Source: CAD feature listing. Evaluate the final solid. Frame: model axes, mm. Face numbers are marked on the shaded views. A direction names the side the tool comes from. Round coordinates to 2 decimals unless told otherwise and drop trailing zeros. Order: outer loops, then holes, each group sorted by start corner. A loop starts at its lowest first (then second) coordinate and runs counter-clockwise, first axis right, second up. Notation, with made-up numbers: (86, 51) -> (98, 51) arc R16 cw to (98, 62) -> close; hole circle Ø2 at (46, 49). An arc over 180 degrees is marked (long way). Answer as CSV lines item,"result". Start each with the question number.
(1) Line query: line 1 along Z through (x, y) = (-8, 6); line 2 along X through (y, z) = (40.5, -2.75); line 3 along Z through (x, y) = (20.5, 46.5). Output: solid intervals per line, ascending. Write a range as from..to.
(2) Section query A-A (x = -17). Output: boundary loops of the cut face in (y, z).
(3) Pull-direction query (Z, two-part tool) for the marked faces 3, 4 and 5; classes: +Z half, -Z half, draft (parallel to the pull), parting line (faces both ways), or undercut.
(4) Section query B-B (z = 5.5). Output: boundary loops of the cut face in (x, y), plus the area to 3 significant figures.
(5) Section query C-C (y = 75.5). Output: boundary loops of the cut face in (x, z) (3 decimals).
(6) Set-up query: the marked faces 1 and 2. Return all of +Z, -Z, +X, -X, +Y, -Y with unobstructed straight access to the full face (end or side cutting, diameter ignored); none if empty.
(7) Contact query for a flat-ended pin moving along its axis: P1, Ø3, axis at y = 50, z = -9, coming from the +X side. Output: stop coordinate, or through.
Solid Edge part; units mm, degrees
sketch "Sketch1" plane through (0, 0, 0) normal (1, 0, 0) x (0, 1, 0)
  line L0 (0, 0) -> (127.0003, 0)
sketch "Sketch2" plane through (0, 0, 0) normal (0, -1, 0) x (1, 0, 0)
  line L0 (25.4001, -6.985) -> (25.4001, 6.985)
  arc A0 (19.6851, 12.7) -> (25.4001, 6.985) centre (19.6851, 6.985) cw
  line L1 (19.6851, 12.7) -> (-19.6851, 12.7)
  arc A1 (-19.6851, 12.7) -> (-25.4001, 6.985) centre (-19.6851, 6.985) ccw
  line L2 (-25.4001, 6.985) -> (-25.4001, -6.985)
  arc A2 (-25.4001, -6.985) -> (-19.6851, -12.7) centre (-19.6851, -6.985) ccw
  line L3 (-19.6851, -12.7) -> (19.6851, -12.7)
  arc A3 (19.6851, -12.7) -> (25.4001, -6.985) centre (19.6851, -6.985) ccw
sweep "Protrusion_1" add profiles "Sketch2" path "Sketch1"
sketch "Sketch3" plane through (0, 0, 0) normal (1, 0, 0) x (0, 1, 0)
  line L0 (0, 0) -> (127.0003, 0)
sketch "Sketch4" plane through (0, 0, 0) normal (0, -1, 0) x (1, 0, 0)
  line L0 (-19.6851, -10.16) -> (19.6851, -10.16)
  arc A0 (19.6851, -10.16) -> (22.8601, -6.985) centre (19.6851, -6.985) ccw
  line L1 (22.8601, -6.985) -> (22.8601, 6.985)
  arc A1 (22.8601, 6.985) -> (19.6851, 10.16) centre (19.6851, 6.985) ccw
  line L2 (19.6851, 10.16) -> (-19.6851, 10.16)
  arc A2 (-19.6851, 10.16) -> (-22.8601, 6.985) centre (-19.6851, 6.985) ccw
  line L3 (-22.8601, 6.985) -> (-22.8601, -6.985)
  arc A3 (-22.8601, -6.985) -> (-19.6851, -10.16) centre (-19.6851, -6.985) ccw
sweep "Cutout_1" cut profiles "Sketch4" path "Sketch3"
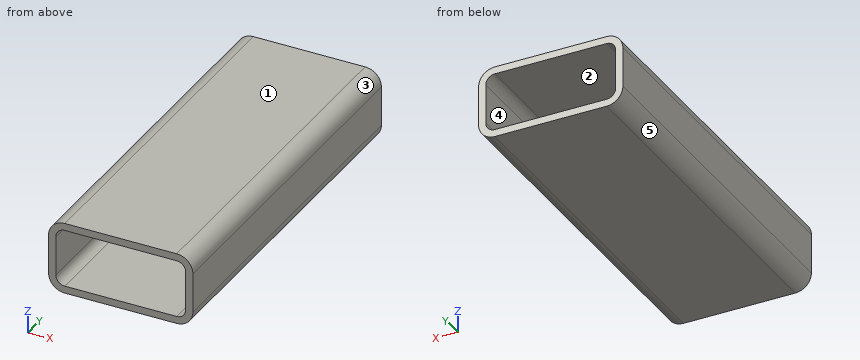
Answer block:
1,line 1,"-12.7..-10.16, 10.16..12.7"
1,line 2,"-25.4..-22.86, 22.86..25.4"
1,line 3,"-12.64..-10.05, 10.05..12.64"
2,outline,"(0, -12.7) -> (127, -12.7) -> (127, -10.16) -> (0, -10.16) -> close; (0, 10.16) -> (127, 10.16) -> (127, 12.7) -> (0, 12.7) -> close"
3,face 3,"+Z half"
3,face 4,"undercut"
3,face 5,"-Z half"
4,outline,"(-25.4, 0) -> (-22.86, 0) -> (-22.86, 127) -> (-25.4, 127) -> close; (22.86, 0) -> (25.4, 0) -> (25.4, 127) -> (22.86, 127) -> close"
4,area,"645 mm2"
5,outline,"(-25.4, -6.985) arc R5.715 ccw to (-19.685, -12.7) -> (19.685, -12.7) arc R5.715 ccw to (25.4, -6.985) -> (25.4, 6.985) arc R5.715 ccw to (19.685, 12.7) -> (-19.685, 12.7) arc R5.715 ccw to (-25.4, 6.985) -> close; hole (-22.86, -6.985) arc R3.175 ccw to (-19.685, -10.16) -> (19.685, -10.16) arc R3.175 ccw to (22.86, -6.985) -> (22.86, 6.985) arc R3.175 ccw to (19.685, 10.16) -> (-19.685, 10.16) arc R3.175 ccw to (-22.86, 6.985) -> close"
6,face 1,"+Z, +X, -X, +Y, -Y"
6,face 2,"+Y, -Y"
7,P1,"x = 25.38"
